Could you check a few things on this model? Use its own coordinates, in mm. A direction names the side the tool comes from. Give positions to 0.01 mm unless a question says otherwise; leave off trailing zeros. Answer in a Markdown table with one row per item. Add a question column.
```python
from build123d import *

# Parameters (mm, degrees)
SKETCH1_W               = 250
SKETCH1_H               = 250
BOSS_EXTRUDE1_DEPTH     = 20
CUT_EXTRUDE1_DEPTH      = 281.223125384
CUT_EXTRUDE2_DEPTH      = 184.527379594
CUT_EXTRUDE2_DEPTH_BACK = 184.527379594
SKETCH3_R               = 12.5
CUT_EXTRUDE3_DEPTH      = 261.116460281
CUT_EXTRUDE5_DEPTH      = 261.116460289


with BuildPart() as part:
    # Sketch1 → Boss-Extrude1 (new body)
    with BuildSketch(Plane(origin=(0, 0, 0), x_dir=(1, 0, 0), z_dir=(0, 1, 0))):
        Rectangle(SKETCH1_W, SKETCH1_H)
    extrude(amount=BOSS_EXTRUDE1_DEPTH)

    # Sketch2 → Cut-Extrude1 (cut, through all)
    with BuildSketch(Plane(origin=(125, 0, 0), x_dir=(0, 0, -1), z_dir=(1, 0, 0))):
        Polygon((125, 2.822268508), (125, 0), (98.147908825, 0), align=None)
    extrude(amount=-CUT_EXTRUDE1_DEPTH, mode=Mode.SUBTRACT)

    # Sketch3 → Cut-Extrude2 (cut, two sides: drawn at the far end of the back side and taken through both)
    with BuildSketch(Plane(origin=(0, -20.175156681, -3.23125924), x_dir=(1, 0, 0), z_dir=(0, -0.9781476007338071, -0.20791169081775307)).offset(-CUT_EXTRUDE2_DEPTH_BACK)):
        with Locations(Location((0, -110.463189586, 0), (0, 0, 270))):
            Circle(SKETCH3_R)
    extrude(amount=CUT_EXTRUDE2_DEPTH + CUT_EXTRUDE2_DEPTH_BACK, mode=Mode.SUBTRACT)

    # Sketch4 → Cut-Extrude3 (cut, through all)
    with BuildSketch(Plane(origin=(56.770360605, 0, -59.986780379), x_dir=(0.7660444431189859, 0, 0.6427876096865301), z_dir=(-0.6427876096865301, 0, 0.7660444431189859))):
        with BuildLine():
            Line((-84.785520804, 20), (-63.4313643, 20))
            ThreePointArc((-63.4313643, 20), (-61.650530379, 14.524902088), (-62.512612953, 8.832373631))
            Line((-62.512612953, 8.832373631), (-70.344986584, 1))
            Line((-70.344986584, 1), (-77.871898519, 1))
            Line((-77.871898519, 1), (-85.704272151, 8.832373631))
            ThreePointArc((-85.704272151, 8.832373631), (-86.566354725, 14.524902088), (-84.785520804, 20))
        make_face()
    extrude(amount=CUT_EXTRUDE3_DEPTH, mode=Mode.SUBTRACT)

    # Sketch9 → Cut-Extrude5 (cut, through all)
    with BuildSketch(Plane(origin=(-56.770360605, 0, -59.986780379), x_dir=(-0.766044443118977, 0, 0.6427876096865405), z_dir=(-0.6427876096865405, 0, -0.766044443118977))):
        with BuildLine():
            Line((-63.4313643, 20), (-84.785520804, 20))
            ThreePointArc((-84.785520804, 20), (-86.566354725, 14.524902088), (-85.704272151, 8.832373631))
            Line((-85.704272151, 8.832373631), (-77.871898519, 1))
            Line((-77.871898519, 1), (-70.344986584, 1))
            Line((-70.344986584, 1), (-62.512612953, 8.832373631))
            ThreePointArc((-62.512612953, 8.832373631), (-61.650530379, 14.524902088), (-63.4313643, 20))
        make_face()
    extrude(amount=-CUT_EXTRUDE5_DEPTH, mode=Mode.SUBTRACT)


solid = part.part
```
Item 1: For faces 5 (the face through (66, 1, -29)), 6 (the face through (-2, 20, 39)), 7 (the face through (61.03, 14.44, -15.5)), which set-ups out of +Z, -Z, +X, -X, +Y, -Y let a thin tool reach every point of the face, with its end or its side?
Item 2: If we mould it in two halves opening along Z, with no side actions, what happens to faces 1 (the face through (-2, 10, 125)), 2 (the face through (26, 20, -101)), 3 (the face through (62.459, 4.861, -21.324)), 4 (the face through (-2, 11, -125))? For each: +Z half, -Z half, draft (parallel to the pull), parting line (faces both ways), or undercut.
Item 3: I need wall thicknesses on L1, parallel to X at y = 18, z = -13; L2, parallel to X at y = 14, z = -45; L3, parallel to Y at x = -79.5, z = -18. Which ranges of each line are inside material? Lowest first, please.
Values found:
| question | item | result |
|---|---|---|
| 1 | face 5 | +Y |
| 1 | face 6 | +Z, -Z, +X, -X, +Y |
| 1 | face 7 | none |
| 2 | face 1 | +Z half |
| 2 | face 2 | draft |
| 2 | face 3 | undercut |
| 2 | face 4 | -Z half |
| 3 | L1 | -125 to -94.62, -64.17 to 64.17, 94.62 to 125 |
| 3 | L2 | -125 to -68.85, -36.24 to 36.24, 68.85 to 125 |
| 3 | L3 | 0 to 1 |
